Part print with two shaded views. Sizes in mm from the minimum x, y, z corner. Coordinates: 2 decimals unless noted, no trailing zeros. Write each loop counter-clockwise with the first axis right and the second up, starting at its lowest first coordinate (ties: lowest second). Pieces come first, ordered by that corner, then holes. Notation, with made-up numbers: (42.5, 63.5) - (99.5, 63.5) arc R25 ccw to (99.5, 94.5) - close; hole circle Ø8 at (25, 49.5). An arc over 180 degrees is marked (long way). One line per question, with ' | ' between items. Start each with the question number.
1. Band-saw the part on B-B, the plane y = 4. Write the cut outline in (x, z), then the cut area to 3 significant figures.
2. Probe line 1 (Z direction, x = 87.5, y = 3.5); line 2 (Z direction, x = 51, y = 0.2); line 3 (X direction, y = 4.05, z = 11). List the from-to ranges inside material, lowest first.
3. Band-saw the part on C-C, the plane z = 29. Write the cut outline in (x, y).
4. Flat gauge pins, fed straight in: P1, Ø0.6, axis at x = 36.5, y = 4, coming from the -Z side; P2, Ø4, axis at x = 71.5, z = 99.5, coming from the -Y side; P3, Ø1.5, axis at y = 2.5, z = 75.5, coming from the +X side. Where does each tip first touch, or does it go through?
5. Band-saw the part on A-A, the plane x = 56. Write the cut outline in (y, z).
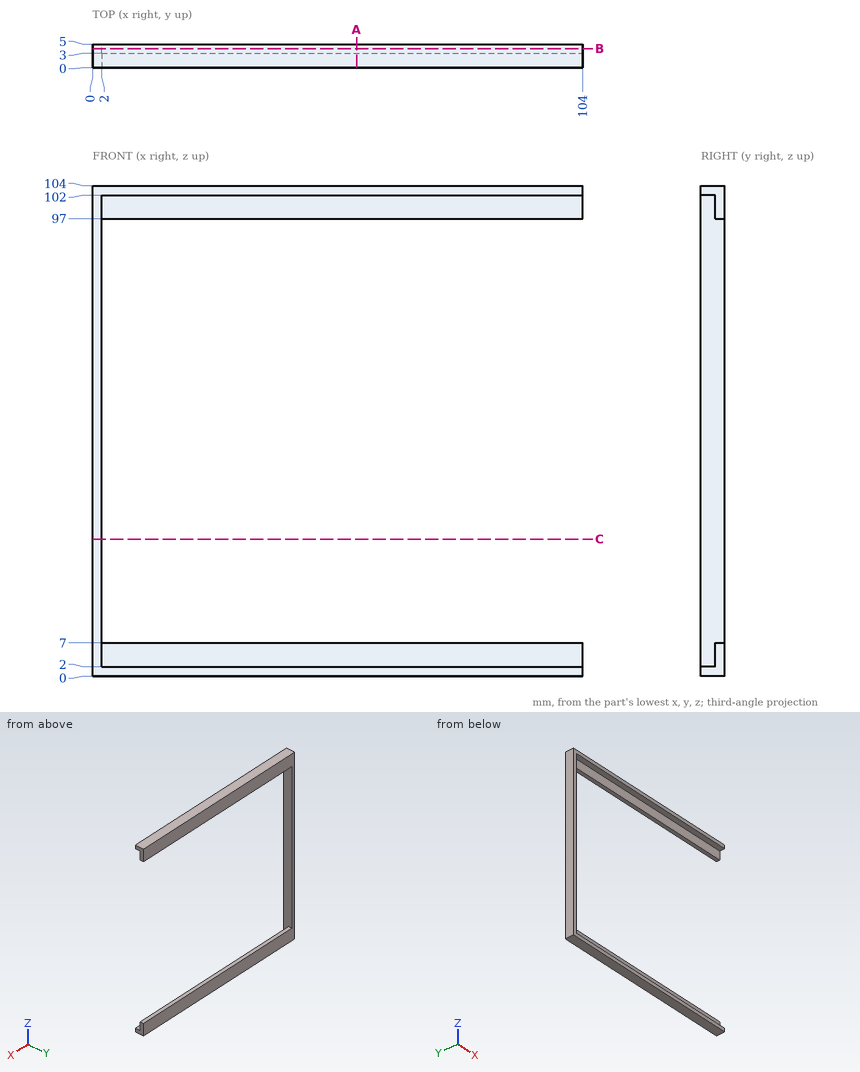
Filled in:
1) outline: (0, 0) - (104, 0) - (104, 7) - (2, 7) - (2, 97) - (104, 97) - (104, 104) - (0, 104) - close | area: 1,640 mm²
2) line 1: z = 0 to 7, 97 to 104 | line 2: z = 0 to 2, 102 to 104 | line 3: x = 0 to 2
3) outline: (0, 0) - (2, 0) - (2, 5) - (0, 5) - close
4) P1: stops at z = 0 | P2: stops at y = 3 | P3: stops at x = 2
5) outline: (0, 0) - (5, 0) - (5, 7) - (3, 7) - (3, 2) - (0, 2) - close; (0, 102) - (3, 102) - (3, 97) - (5, 97) - (5, 104) - (0, 104) - close
